Verification items for the finished model (mm, model axes). A direction names the side the tool comes from. Coordinates: 2 decimals unless noted, no trailing zeros. Write each loop counter-clockwise with the first axis right and the second up, starting at its lowest first coordinate (ties: lowest second). Pieces come first, ordered by that corner, then holes. Notation, with made-up numbers: (34, 29) -> (70, 29) arc R6 cw to (70, 34) -> close; hole circle Ø2 at (58.25, 84). An arc over 180 degrees is marked (long way). Use CSV: the item, a comma, the result in double quotes.
```python
from build123d import *

# Parameters (mm, degrees)
PAD_DEPTH       = 10
POCKET_DEPTH    = 6
POCKET001_DEPTH = 2


with BuildPart() as part:
    # Sketch → Pad (new body)
    with BuildSketch(Plane.XY):
        with BuildLine():
            Line((-18.212601, -22), (-3.787399, -22))
            ThreePointArc((-3.787399, -22), (-1.109303, -20.890697), (0, -18.212601))
            Line((0, -18.212601), (0, -3.787399))
            ThreePointArc((0, -3.787399), (-1.109303, -1.109303), (-3.787399, 0))
            Line((-3.787399, 0), (-18.212601, 0))
            ThreePointArc((-18.212601, 0), (-20.890697, -1.109303), (-22, -3.787399))
            Line((-22, -3.787399), (-22, -18.212601))
            ThreePointArc((-22, -18.212601), (-20.890697, -20.890697), (-18.212601, -22))
        make_face()
    extrude(amount=PAD_DEPTH)

    # Sketch001 (on Face10 of Pad) → Pocket (cut)
    with BuildSketch(Plane.XY.offset(10)):
        Polygon((-4, -4), (-4, -24), (-5.9, -24), (-5.9, -5.9), (-24, -5.9), (-24, -4), align=None)
    extrude(amount=-POCKET_DEPTH, mode=Mode.SUBTRACT)

    # Sketch002 (on Face2 of Pocket) → Pocket001 (cut)
    with BuildSketch(Plane(origin=(0, 0, 0), x_dir=(1, 0, 0), z_dir=(0, 0, -1))):
        with BuildLine():
            Line((-21.5, 17.5), (-21.5, 4.5))
            ThreePointArc((-21.5, 4.5), (-20.328427, 1.671573), (-17.5, 0.5))
            Line((-17.5, 0.5), (-4.5, 0.5))
            ThreePointArc((-4.5, 0.5), (-1.671573, 1.671573), (-0.5, 4.5))
            Line((-0.5, 4.5), (-0.5, 17.5))
            ThreePointArc((-0.5, 17.5), (-1.671573, 20.328427), (-4.5, 21.5))
            Line((-4.5, 21.5), (-17.5, 21.5))
            ThreePointArc((-17.5, 21.5), (-20.328427, 20.328427), (-21.5, 17.5))
        make_face()
    extrude(amount=-POCKET001_DEPTH, mode=Mode.SUBTRACT)


solid = part.part
```
1) Cross-section at A-A (z = 4.5). Record the boundary of the cut face in (x, y), plus the area to 3 significant figures.
Return value:
outline,"(-22, -18.21) arc R3.79 ccw to (-18.21, -22) -> (-5.9, -22) -> (-5.9, -5.9) -> (-22, -5.9) -> close; (-22, -4) -> (-4, -4) -> (-4, -22) -> (-3.79, -22) arc R3.79 ccw to (0, -18.21) -> (0, -3.79) arc R3.79 ccw to (-3.79, 0) -> (-18.21, 0) arc R3.79 ccw to (-22, -3.79) -> close"
area,"407 mm2"
2) Set-up check for faces 4 (the flat face through (-4, -13, 7)), 5 (the cylindrical face through (-20.297, -20.359, 0.986)), 6 (the flat face through (-14, -14, 10)): record each of +Z, -Z, +X, -X, +Y, -Y from which the full face is reachable in a straight line by a thin tool's end or side.
Return value:
face 4,"+Z, -Y"
face 5,"-Z"
face 6,"+Z, +X, -X, +Y, -Y"
3) Cross-section at D-D (y = -2.5). Record the boundary of the cut face in (x, z), plus the area to 3 significant figures.
Return value:
outline,"(-21.77, 0) -> (-20.96, 0) -> (-20.96, 2) -> (-1.04, 2) -> (-1.04, 0) -> (-0.23, 0) -> (-0.23, 10) -> (-21.77, 10) -> close"
area,"176 mm2"
4) Cross-section at B-B (y = -14.75). Record the boundary of the cut face in (x, z).
Return value:
outline,"(-22, 0) -> (-21.5, 0) -> (-21.5, 2) -> (-0.5, 2) -> (-0.5, 0) -> (0, 0) -> (0, 10) -> (-4, 10) -> (-4, 4) -> (-5.9, 4) -> (-5.9, 10) -> (-22, 10) -> close"
5) Mould release check, pull along X, two halves, no side actions. Record for faces 1 (the flat face through (0, -11, 5)), 2 (the flat face through (-3.8, -8.4, 10)), 3 (the flat face through (-11, -11, 2)): released by +X, released by -X, zero draft, split by the parting line, or undercut.
Return value:
face 1,"released by +X"
face 2,"zero draft"
face 3,"undercut"
6) Scan lines: L1, parallel to Y at x = -16, z = 1.5; L2, parallel to Y at x = -6.25, z = 5.25. Record each from-to range of solid material in increasing order.
Return value:
L1,"-22 to -21.5, -0.5 to 0"
L2,"-22 to -5.9, -4 to 0"
7) Gauge pin test, flat end, axial feed: pin 1 (5 mm diameter, centred on x = -19.5, z = 5.5, fed in from +Y). Record the tip position at first contact, or that the pin passes through.
Return value:
pin 1,"y = 0"
